Can you work these out from the model? Positions are in its coordinate system, mm. A direction names the side the tool comes from. Give positions to 0.01 mm unless a question says otherwise; leave off trailing zeros. Write each loop counter-clockwise with the first axis right and the second up, starting at its lowest first coordinate (ties: lowest second). Pieces come first, ordered by that corner, then holes.
1. Suppose I cut it at A-A (y = -53.5). Please give me the cut outline in (x, z).
2. On a 3-axis mill with a long thin cutter (end or side, diameter ignored), from which of +Z, -Z, +X, -X, +Y, -Y can I reach the whole of each face in a straight line? I mean faces 1 (the cylindrical face through (-27.305, -56.252, -4.93)), 2 (the cylindrical face through (-16.01, -53.3, -4.93)), 3 (the cylindrical face through (-24.557, -71.132, -4.93)), 4 (the flat face through (-13.86, -60.9, -6.55)). Say none if no direction works.
3. If I drill on probe 1 along Y at (x, z) = (-28.5, -3.5); probe 2 along Y at (x, z) = (-10.5, -7.75); probe 3 along Y at (x, z) = (-16, -3.5), over which ranges is the centre line in solid material (lowest first)?
4. I'm going to push flat-ended pins straight in: pin 1 (5 mm diameter, centred on x = -19.63, y = -62.55, fed in from -Z); pin 2 (5 mm diameter, centred on y = -63.5, z = -2.5, fed in from +X). Where does each tip first touch, or does it pass through?
5. Thinking about a two-plate mould opening in Y: for faces 5 (the flat face through (-15, -67, -10)), 6 (the cylindrical face through (-19.046, -52.636, -4.93)), 7 (the cylindrical face through (-14.654, -55.351, -4.93)), which applies, pulls with the +Y half, pulls with the -Y half, needs draft (parallel to the pull), parting line crosses it, or undercut?
```python
from build123d import *

# Parameters (mm, degrees)
SKETCH1_R           = 2.25
BOSS_EXTRUDE1_DEPTH = 10
CUT_EXTRUDE1_DEPTH  = 7


with BuildPart() as part:
    # Sketch1 → Boss-Extrude1 (new body)
    with BuildSketch(Plane.XY):
        with BuildLine():
            ThreePointArc((-30.571614903, -61.443860954), (-29.524113514, -61.972609686), (-28.368252904, -62.174650848))
            ThreePointArc((-28.368252904, -62.174650848), (-28.373609105, -62.764315084), (-28.339231944, -63.353000748))
            ThreePointArc((-28.339231944, -63.353000748), (-29.483745303, -63.611696612), (-30.503947952, -64.19136974))
            ThreePointArc((-30.503947952, -64.19136974), (-30.446172213, -64.536660067), (-30.377437772, -64.879936957))
            ThreePointArc((-30.377437772, -64.879936957), (-29.217812407, -65.059111153), (-28.056089489, -64.894083145))
            ThreePointArc((-28.056089489, -64.894083145), (-27.878967269, -65.456542317), (-27.664358771, -66.005792526))
            ThreePointArc((-27.664358771, -66.005792526), (-28.672914241, -66.605500992), (-29.464055771, -67.472062854))
            ThreePointArc((-29.464055771, -67.472062854), (-29.302407199, -67.782599785), (-29.130958468, -68.087835397))
            ThreePointArc((-29.130958468, -68.087835397), (-27.972721336, -67.899896238), (-26.918853644, -67.383953152))
            ThreePointArc((-26.918853644, -67.383953152), (-26.57659096, -67.864149836), (-26.202758501, -68.320200154))
            ThreePointArc((-26.202758501, -68.320200154), (-26.976631645, -69.202217578), (-27.46126961, -70.270843062))
            ThreePointArc((-27.46126961, -70.270843062), (-27.211571493, -70.516229077), (-26.954191069, -70.753544823))
            ThreePointArc((-26.954191069, -70.753544823), (-25.910718491, -70.216889105), (-25.067865938, -69.400535044))
            ThreePointArc((-25.067865938, -69.400535044), (-24.593965845, -69.751464244), (-24.09750275, -70.069673287))
            ThreePointArc((-24.09750275, -70.069673287), (-24.560941474, -71.147661659), (-24.691636133, -72.313746256))
            ThreePointArc((-24.691636133, -72.313746256), (-24.378330663, -72.469961264), (-24.060212735, -72.616127025))
            ThreePointArc((-24.060212735, -72.616127025), (-23.233647078, -71.783286348), (-22.684313942, -70.746431736))
            ThreePointArc((-22.684313942, -70.746431736), (-22.125165085, -70.933742055), (-21.554668621, -71.082961306))
            ThreePointArc((-21.554668621, -71.082961306), (-21.662308312, -72.251399614), (-21.426266363, -73.400798839))
            ThreePointArc((-21.426266363, -73.400798839), (-21.080022062, -73.452551425), (-20.732306229, -73.493259479))
            ThreePointArc((-20.732306229, -73.493259479), (-20.203557497, -72.44575809), (-20.001516335, -71.289897481))
            ThreePointArc((-20.001516335, -71.289897481), (-19.411852099, -71.295253682), (-18.823166434, -71.26087652))
            ThreePointArc((-18.823166434, -71.26087652), (-18.56447057, -72.40538988), (-17.984797442, -73.425592529))
            ThreePointArc((-17.984797442, -73.425592529), (-17.639507115, -73.36781679), (-17.296230226, -73.299082349))
            ThreePointArc((-17.296230226, -73.299082349), (-17.11705603, -72.139456983), (-17.282084037, -70.977734066))
            ThreePointArc((-17.282084037, -70.977734066), (-16.719624866, -70.800611845), (-16.170374656, -70.586003347))
            ThreePointArc((-16.170374656, -70.586003347), (-15.57066619, -71.594558818), (-14.704104328, -72.385700347))
            ThreePointArc((-14.704104328, -72.385700347), (-14.393567398, -72.224051775), (-14.088331786, -72.052603044))
            ThreePointArc((-14.088331786, -72.052603044), (-14.276270944, -70.894365913), (-14.79221403, -69.840498221))
            ThreePointArc((-14.79221403, -69.840498221), (-14.312017346, -69.498235536), (-13.855967028, -69.124403077))
            ThreePointArc((-13.855967028, -69.124403077), (-12.973949604, -69.898276222), (-11.905324121, -70.382914186))
            ThreePointArc((-11.905324121, -70.382914186), (-11.659938105, -70.13321607), (-11.422622359, -69.875835646))
            ThreePointArc((-11.422622359, -69.875835646), (-11.959278077, -68.832363068), (-12.775632138, -67.989510514))
            ThreePointArc((-12.775632138, -67.989510514), (-12.424702939, -67.515610422), (-12.106493895, -67.019147327))
            ThreePointArc((-12.106493895, -67.019147327), (-11.028505523, -67.48258605), (-9.862420926, -67.61328071))
            ThreePointArc((-9.862420926, -67.61328071), (-9.706205919, -67.29997524), (-9.560040157, -66.981857312))
            ThreePointArc((-9.560040157, -66.981857312), (-10.392880835, -66.155291654), (-11.429735447, -65.605958519))
            ThreePointArc((-11.429735447, -65.605958519), (-11.242425127, -65.046809661), (-11.093205876, -64.476313197))
            ThreePointArc((-11.093205876, -64.476313197), (-9.924767569, -64.583952889), (-8.775368344, -64.347910939))
            ThreePointArc((-8.775368344, -64.347910939), (-8.723615758, -64.001666638), (-8.682907704, -63.653950805))
            ThreePointArc((-8.682907704, -63.653950805), (-9.730409092, -63.125202073), (-10.886269702, -62.923160911))
            ThreePointArc((-10.886269702, -62.923160911), (-10.880913501, -62.333496675), (-10.915290662, -61.744811011))
            ThreePointArc((-10.915290662, -61.744811011), (-9.770777303, -61.486115147), (-8.750574654, -60.906442019))
            ThreePointArc((-8.750574654, -60.906442019), (-8.808350393, -60.561151691), (-8.877084834, -60.217874802))
            ThreePointArc((-8.877084834, -60.217874802), (-10.036710199, -60.038700606), (-11.198433117, -60.203728614))
            ThreePointArc((-11.198433117, -60.203728614), (-11.375555337, -59.641269442), (-11.590163835, -59.092019232))
            ThreePointArc((-11.590163835, -59.092019232), (-10.581608365, -58.492310767), (-9.790466835, -57.625748905))
            ThreePointArc((-9.790466835, -57.625748905), (-9.952115407, -57.315211974), (-10.123564138, -57.009976362))
            ThreePointArc((-10.123564138, -57.009976362), (-11.28180127, -57.19791552), (-12.335668962, -57.713858607))
            ThreePointArc((-12.335668962, -57.713858607), (-12.677931646, -57.233661923), (-13.051764106, -56.777611605))
            ThreePointArc((-13.051764106, -56.777611605), (-12.277890961, -55.89559418), (-11.793252996, -54.826968697))
            ThreePointArc((-11.793252996, -54.826968697), (-12.042951113, -54.581582682), (-12.300331537, -54.344266935))
            ThreePointArc((-12.300331537, -54.344266935), (-13.343804115, -54.880922654), (-14.186656669, -55.697276715))
            ThreePointArc((-14.186656669, -55.697276715), (-14.660556761, -55.346347515), (-15.157019856, -55.028138471))
            ThreePointArc((-15.157019856, -55.028138471), (-14.693581132, -53.9501501), (-14.562886473, -52.784065503))
            ThreePointArc((-14.562886473, -52.784065503), (-14.876191943, -52.627850495), (-15.194309871, -52.481684734))
            ThreePointArc((-15.194309871, -52.481684734), (-16.020875528, -53.314525411), (-16.570208664, -54.351380023))
            ThreePointArc((-16.570208664, -54.351380023), (-17.129357521, -54.164069704), (-17.699853985, -54.014850452))
            ThreePointArc((-17.699853985, -54.014850452), (-17.592214294, -52.846412145), (-17.828256244, -51.69701292))
            ThreePointArc((-17.828256244, -51.69701292), (-18.174500544, -51.645260334), (-18.522216377, -51.60455228))
            ThreePointArc((-18.522216377, -51.60455228), (-19.050965109, -52.652053668), (-19.253006271, -53.807914278))
            ThreePointArc((-19.253006271, -53.807914278), (-19.842670508, -53.802558077), (-20.431356172, -53.836935239))
            ThreePointArc((-20.431356172, -53.836935239), (-20.690052036, -52.692421879), (-21.269725164, -51.67221923))
            ThreePointArc((-21.269725164, -51.67221923), (-21.615015491, -51.729994969), (-21.95829238, -51.79872941))
            ThreePointArc((-21.95829238, -51.79872941), (-22.137466577, -52.958354776), (-21.972438569, -54.120077693))
            ThreePointArc((-21.972438569, -54.120077693), (-22.53489774, -54.297199913), (-23.08414795, -54.511808411))
            ThreePointArc((-23.08414795, -54.511808411), (-23.683856416, -53.503252941), (-24.550418278, -52.712111412))
            ThreePointArc((-24.550418278, -52.712111412), (-24.860955208, -52.873759984), (-25.16619082, -53.045208714))
            ThreePointArc((-25.16619082, -53.045208714), (-24.978251662, -54.203445846), (-24.462308576, -55.257313538))
            ThreePointArc((-24.462308576, -55.257313538), (-24.94250526, -55.599576222), (-25.398555578, -55.973408682))
            ThreePointArc((-25.398555578, -55.973408682), (-26.280573002, -55.199535537), (-27.349198485, -54.714897573))
            ThreePointArc((-27.349198485, -54.714897573), (-27.594584501, -54.964595689), (-27.831900247, -55.221976113))
            ThreePointArc((-27.831900247, -55.221976113), (-27.295244529, -56.265448691), (-26.478890468, -57.108301245))
            ThreePointArc((-26.478890468, -57.108301245), (-26.829819667, -57.582201337), (-27.148028711, -58.078664432))
            ThreePointArc((-27.148028711, -58.078664432), (-28.226017083, -57.615225709), (-29.39210168, -57.484531049))
            ThreePointArc((-29.39210168, -57.484531049), (-29.548316687, -57.797836519), (-29.694482449, -58.115954447))
            ThreePointArc((-29.694482449, -58.115954447), (-28.861641771, -58.942520105), (-27.824787159, -59.49185324))
            ThreePointArc((-27.824787159, -59.49185324), (-28.012097479, -60.051002097), (-28.16131673, -60.621498562))
            ThreePointArc((-28.16131673, -60.621498562), (-29.329755037, -60.51385887), (-30.479154262, -60.74990082))
            ThreePointArc((-30.479154262, -60.74990082), (-30.530906848, -61.096145121), (-30.571614903, -61.443860954))
        make_face()
        with Locations((-19.627261303, -62.548905879)):
            Circle(SKETCH1_R, mode=Mode.SUBTRACT)
    extrude(amount=-BOSS_EXTRUDE1_DEPTH)

    # Sketch2 → Cut-Extrude1 (cut)
    with BuildSketch(Plane(origin=(0, 0, -10), x_dir=(-1, 0, 0), z_dir=(0, 0, -1))):
        Polygon((24.400288017, -67.570680067), (17.664790642, -69.19335536), (12.891763928, -64.171581173), (14.854234589, -57.527131692), (21.589731964, -55.904456399), (26.362758678, -60.926230586), align=None)
    extrude(amount=-CUT_EXTRUDE1_DEPTH, mode=Mode.SUBTRACT)


solid = part.part
```
Checks:
1. outline: (-25.13, -10) - (-23.69, -10) - (-23.69, 0) - (-25.13, 0) - close; (-22.1, -10) - (-20.47, -10) - (-20.47, 0) - (-22.1, 0) - close; (-19.23, -10) - (-17.61, -10) - (-17.61, 0) - (-19.23, 0) - close; (-16.15, -10) - (-14.6, -10) - (-14.6, 0) - (-16.15, 0) - close
2. face 1: +Z, -Z, -X
2. face 2: +Z, -Z, +Y
2. face 3: +Z, -Z
2. face 4: -Z
3. probe 1: y = -68.03 to -66.47, -65 to -63.37, -62.17 to -60.55, -59.18 to -57.55
3. probe 2: y = -67.59 to -66.08, -64.57 to -62.95, -61.69 to -60.06, -58.42 to -57.03
3. probe 3: y = -70.95 to -67.44, -57.25 to -53.29
4. pin 1: stops at z = -3
4. pin 2: stops at x = -8.68
5. face 5: needs draft
5. face 6: pulls with the +Y half
5. face 7: undercut
